```python
from build123d import *

# Parameters (mm, degrees)
SKETCH1_W                       = 65
SKETCH1_H                       = 65
EXTRUDE1_DEPTH                  = 11.7824246
M6X1_0_TAPPED_HOLE1_D           = 5
CBORE_FOR_M4_SBHCS1_D           = 4.8
CBORE_FOR_M4_SBHCS1_CBORE_D     = 8.6
CBORE_FOR_M4_SBHCS1_CBORE_DEPTH = 8.2


with BuildPart() as part:
    # Sketch1 → Extrude1 (new body)
    with BuildSketch(Plane(origin=(0, 0, 0), x_dir=(1, 0, 0), z_dir=(0, 1, 0))):
        Rectangle(SKETCH1_W, SKETCH1_H)
    extrude(amount=EXTRUDE1_DEPTH)

    # M6x1.0 Tapped Hole1 (through all)
    with Locations(Plane(origin=(0, 11.7824246, 0), x_dir=(-1, 0, 0), z_dir=(0, 1, 0))):
        with Locations((14, -12.6), (14, 12.6)):
            Hole(M6X1_0_TAPPED_HOLE1_D / 2)

    # CBORE for M4 SBHCS1 (through all)
    with Locations(Plane(origin=(0, 11.7824246, 0), x_dir=(-1, 0, 0), z_dir=(0, 1, 0))):
        with Locations((3.402638838, 13), (-22.597361162, 13), (-22.597361162, -13), (3.402638838, -13)):
            CounterBoreHole(CBORE_FOR_M4_SBHCS1_D / 2, CBORE_FOR_M4_SBHCS1_CBORE_D / 2, CBORE_FOR_M4_SBHCS1_CBORE_DEPTH)


solid = part.part
```
Verification items for the finished model (mm, model axes). A direction names the side the tool comes from. Coordinates: 2 decimals unless noted, no trailing zeros. Order: outer loops, then holes, each group sorted by start corner. A loop starts at its lowest first (then second) coordinate and runs counter-clockwise, first axis right, second up. Notation, with made-up numbers: (68.5, -16) - (100.5, -16) arc R19 ccw to (100.5, -11) - close; hole circle Ø11 at (81.25, -11.75). An arc over 180 degrees is marked (long way). Return JSON: item names as keys, results as strings.
(1) Mould release check, pull along Z, two halves, no side actions. Record for faces 3 (the flat face through (21, 3.582, -15)), 4 (the flat face through (32.5, 6, 0)), 5 (the flat face through (0, 6, -32.5)): pulls with the +Z half, pulls with the -Z half, needs draft (parallel to the pull), parting line crosses it, or undercut.
Filled sheet:
{"face 3": "undercut", "face 4": "needs draft", "face 5": "pulls with the -Z half"}
(2) Section check B-B, the plane y = 1.25. Record the cut outline in (x, z), and give its area (3 significant figures).
Filled sheet:
{"outline": "(-32.5, -32.5) - (32.5, -32.5) - (32.5, 32.5) - (-32.5, 32.5) - close; hole circle Ø5 at (-14, -12.6); hole circle Ø5 at (-14, 12.6); hole circle Ø4.8 at (-3.4, -13); hole circle Ø4.8 at (-3.4, 13); hole circle Ø4.8 at (22.6, -13); hole circle Ø4.8 at (22.6, 13)", "area": "4,110 mm^2"}
(3) Thickness scan on line 1 along Z through (x, y) = (-3.5, 6.75); line 2 along Z through (x, y) = (-14, 2.5). Record the ranges inside material, lowest first.
Filled sheet:
{"line 1": "z = -32.5 to -17.3, -8.7 to 8.7, 17.3 to 32.5", "line 2": "z = -32.5 to -15.1, -10.1 to 10.1, 15.1 to 32.5"}
(4) Go/stop test with a flat-tipped pin: pin 1 (4.5 mm diameter, centred on x = -4, z = 13.5, fed in from +Y). Record where the tip stops, or that it passes through.
Filled sheet:
{"pin 1": "stops at y = 3.58"}
(5) Section check D-D, the plane x = 21.5. Record the cut outline in (y, z), and give its area (3 significant figures).
Filled sheet:
{"outline": "(0, -32.5) - (11.78, -32.5) - (11.78, -17.16) - (3.58, -17.16) - (3.58, -15.13) - (0, -15.13) - close; (0, -10.87) - (3.58, -10.87) - (3.58, -8.84) - (11.78, -8.84) - (11.78, 8.84) - (3.58, 8.84) - (3.58, 10.87) - (0, 10.87) - close; (0, 15.13) - (3.58, 15.13) - (3.58, 17.16) - (11.78, 17.16) - (11.78, 32.5) - (0, 32.5) - close", "area": "599 mm^2"}
(6) Section check C-C, the plane y = 10.5. Record the cut outline in (x, z), and give its area (3 significant figures).
Filled sheet:
{"outline": "(-32.5, -32.5) - (32.5, -32.5) - (32.5, 32.5) - (-32.5, 32.5) - close; hole circle Ø5 at (-14, -12.6); hole circle Ø5 at (-14, 12.6); hole circle Ø8.6 at (-3.4, -13); hole circle Ø8.6 at (-3.4, 13); hole circle Ø8.6 at (22.6, -13); hole circle Ø8.6 at (22.6, 13)", "area": "3,950 mm^2"}
(7) Section check A-A, the plane x = -14. Record the cut outline in (y, z).
Filled sheet:
{"outline": "(0, -32.5) - (11.78, -32.5) - (11.78, -15.1) - (0, -15.1) - close; (0, -10.1) - (11.78, -10.1) - (11.78, 10.1) - (0, 10.1) - close; (0, 15.1) - (11.78, 15.1) - (11.78, 32.5) - (0, 32.5) - close"}
(8) Access from +Z, -Z, +X, -X, +Y, -Y to the whole of each face (thin tool, end or side, straight path). Record for faces 1 (the cylindrical face through (-2.11, 1.77, -10.98)), 2 (the flat face through (21, 3.582, 11)).
Filled sheet:
{"face 1": "+Y, -Y", "face 2": "+Y"}
